The listing builds one solid part. Answer for the finished solid, in the listing's coordinates (mm). A direction names the side the tool comes from. Coordinates: 2 decimals unless noted, no trailing zeros. Order: outer loops, then holes, each group sorted by start corner. A loop starts at its lowest first (then second) coordinate and runs counter-clockwise, first axis right, second up. Notation, with made-up numbers: (63, 61.5) -> (121, 61.5) arc R17 cw to (121, 76.5) -> close; hole circle Ø2 at (-13.5, 76.5). An arc over 180 degrees is marked (long way). Return JSON: item names as keys, results as strings.
from build123d import *

# Parameters (mm, degrees)
SKETCH_1_W          = 73.4
SKETCH_1_H          = 53.4
SKETCH_1_W_2        = 70.4
SKETCH_1_H_2        = 50.4
EXTRUDE_1_DEPTH     = 17
SKETCH_2_W          = 73.4
SKETCH_2_H          = 53.4
EXTRUDE_2_DEPTH     = 1.5
SKETCH_3_W          = 4.5
SKETCH_3_H          = 4.5
EXTRUDE_3_DEPTH     = 10.5
CUT_EXTRUDE_1_REACH = 50.464
SKETCH_4_R          = 2
SKETCH_4_R_2        = 1.7
SKETCH_4_R_3        = 3.75
SKETCH_5_R          = 1
CUT_EXTRUDE_2_DEPTH = 7
SKETCH_6_W          = 71.8
SKETCH_6_H          = 51.8
CUT_EXTRUDE_3_DEPTH = 7
CHAMFER_1_SIZE      = 0.5
CUT_EXTRUDE_4_REACH = 68.988
SKETCH_9_W          = 11
SKETCH_9_H          = 13
CUT_EXTRUDE_5_DEPTH = 0.5


with BuildPart() as part:
    # Эскиз1 → Бобышка-Вытянуть1 (new body)
    with BuildSketch(Plane(origin=(0, 0, 0), x_dir=(1, 0, 0), z_dir=(0, 1, 0))):
        Rectangle(SKETCH_1_W, SKETCH_1_H)
        Rectangle(SKETCH_1_W_2, SKETCH_1_H_2, mode=Mode.SUBTRACT)
    extrude(amount=-EXTRUDE_1_DEPTH)

    # Эскиз2 → Бобышка-Вытянуть2 (add)
    with BuildSketch(Plane(origin=(0, 0, 0), x_dir=(1, 0, 0), z_dir=(0, 1, 0))):
        Rectangle(SKETCH_2_W, SKETCH_2_H)
    extrude(amount=EXTRUDE_2_DEPTH)

    # Эскиз3 → Бобышка-Вытянуть3 (add)
    with BuildSketch(Plane(origin=(0, 0, 0), x_dir=(1, 0, 0), z_dir=(0, 1, 0))):
        with Locations((-32.95, 22.95)):
            Rectangle(SKETCH_3_W, SKETCH_3_H)
        with Locations((32.95, 22.95)):
            Rectangle(SKETCH_3_W, SKETCH_3_H)
        with Locations((-32.95, -22.95)):
            Rectangle(SKETCH_3_W, SKETCH_3_H)
        with Locations((32.95, -22.95)):
            Rectangle(SKETCH_3_W, SKETCH_3_H)
    extrude(amount=-EXTRUDE_3_DEPTH)

    # Эскиз4 → Вырез-Вытянуть1 (cut, up to next)
    with BuildSketch(Plane(origin=(0, 0, 0), x_dir=(1, 0, 0), z_dir=(0, 1, 0)), mode=Mode.PRIVATE) as cut_extrude_1_sk1:
        with Locations(Location((-25.4, -9, 0), (0, 0, 270))):
            Circle(SKETCH_4_R)
    cut_extrude_1_tool1 = extrude(cut_extrude_1_sk1.sketch, amount=CUT_EXTRUDE_1_REACH, mode=Mode.PRIVATE) & part.part
    # Эскиз4 → Вырез-Вытянуть1 (cut, up to next)
    with BuildSketch(Plane(origin=(0, 0, 0), x_dir=(1, 0, 0), z_dir=(0, 1, 0)), mode=Mode.PRIVATE) as cut_extrude_1_sk2:
        with Locations(Location((-12.7, -9, 0), (0, 0, 270))):
            Circle(SKETCH_4_R)
    cut_extrude_1_tool2 = extrude(cut_extrude_1_sk2.sketch, amount=CUT_EXTRUDE_1_REACH, mode=Mode.PRIVATE) & part.part
    # Эскиз4 → Вырез-Вытянуть1 (cut, up to next)
    with BuildSketch(Plane(origin=(0, 0, 0), x_dir=(1, 0, 0), z_dir=(0, 1, 0)), mode=Mode.PRIVATE) as cut_extrude_1_sk3:
        with Locations(Location((0, -9, 0), (0, 0, 270))):
            Circle(SKETCH_4_R)
    cut_extrude_1_tool3 = extrude(cut_extrude_1_sk3.sketch, amount=CUT_EXTRUDE_1_REACH, mode=Mode.PRIVATE) & part.part
    # Эскиз4 → Вырез-Вытянуть1 (cut, up to next)
    with BuildSketch(Plane(origin=(0, 0, 0), x_dir=(1, 0, 0), z_dir=(0, 1, 0)), mode=Mode.PRIVATE) as cut_extrude_1_sk4:
        with Locations(Location((12.7, -9, 0), (0, 0, 270))):
            Circle(SKETCH_4_R)
    cut_extrude_1_tool4 = extrude(cut_extrude_1_sk4.sketch, amount=CUT_EXTRUDE_1_REACH, mode=Mode.PRIVATE) & part.part
    # Эскиз4 → Вырез-Вытянуть1 (cut, up to next)
    with BuildSketch(Plane(origin=(0, 0, 0), x_dir=(1, 0, 0), z_dir=(0, 1, 0)), mode=Mode.PRIVATE) as cut_extrude_1_sk5:
        with Locations(Location((25.4, -9, 0), (0, 0, 270))):
            Circle(SKETCH_4_R)
    cut_extrude_1_tool5 = extrude(cut_extrude_1_sk5.sketch, amount=CUT_EXTRUDE_1_REACH, mode=Mode.PRIVATE) & part.part
    # Эскиз4 → Вырез-Вытянуть1 (cut, up to next)
    with BuildSketch(Plane(origin=(0, 0, 0), x_dir=(1, 0, 0), z_dir=(0, 1, 0)), mode=Mode.PRIVATE) as cut_extrude_1_sk6:
        with Locations(Location((-25.4, 6, 0), (0, 0, 270))):
            Circle(SKETCH_4_R_2)
    cut_extrude_1_tool6 = extrude(cut_extrude_1_sk6.sketch, amount=CUT_EXTRUDE_1_REACH, mode=Mode.PRIVATE) & part.part
    # Эскиз4 → Вырез-Вытянуть1 (cut, up to next)
    with BuildSketch(Plane(origin=(0, 0, 0), x_dir=(1, 0, 0), z_dir=(0, 1, 0)), mode=Mode.PRIVATE) as cut_extrude_1_sk7:
        with Locations(Location((-17.78, 6, 0), (0, 0, 270))):
            Circle(SKETCH_4_R_2)
    cut_extrude_1_tool7 = extrude(cut_extrude_1_sk7.sketch, amount=CUT_EXTRUDE_1_REACH, mode=Mode.PRIVATE) & part.part
    # Эскиз4 → Вырез-Вытянуть1 (cut, up to next)
    with BuildSketch(Plane(origin=(0, 0, 0), x_dir=(1, 0, 0), z_dir=(0, 1, 0)), mode=Mode.PRIVATE) as cut_extrude_1_sk8:
        with Locations(Location((-10.16, 6, 0), (0, 0, 270))):
            Circle(SKETCH_4_R_2)
    cut_extrude_1_tool8 = extrude(cut_extrude_1_sk8.sketch, amount=CUT_EXTRUDE_1_REACH, mode=Mode.PRIVATE) & part.part
    # Эскиз4 → Вырез-Вытянуть1 (cut, up to next)
    with BuildSketch(Plane(origin=(0, 0, 0), x_dir=(1, 0, 0), z_dir=(0, 1, 0)), mode=Mode.PRIVATE) as cut_extrude_1_sk9:
        with Locations(Location((21.5, 8, 0), (0, 0, 270))):
            Circle(SKETCH_4_R_3)
    cut_extrude_1_tool9 = extrude(cut_extrude_1_sk9.sketch, amount=CUT_EXTRUDE_1_REACH, mode=Mode.PRIVATE) & part.part
    add(cut_extrude_1_tool1.solids().sort_by_distance((-25.4, 0, 9))[0], mode=Mode.SUBTRACT)
    add(cut_extrude_1_tool2.solids().sort_by_distance((-12.7, 0, 9))[0], mode=Mode.SUBTRACT)
    add(cut_extrude_1_tool3.solids().sort_by_distance((0, 0, 9))[0], mode=Mode.SUBTRACT)
    add(cut_extrude_1_tool4.solids().sort_by_distance((12.7, 0, 9))[0], mode=Mode.SUBTRACT)
    add(cut_extrude_1_tool5.solids().sort_by_distance((25.4, 0, 9))[0], mode=Mode.SUBTRACT)
    add(cut_extrude_1_tool6.solids().sort_by_distance((-25.4, 0, -6))[0], mode=Mode.SUBTRACT)
    add(cut_extrude_1_tool7.solids().sort_by_distance((-17.78, 0, -6))[0], mode=Mode.SUBTRACT)
    add(cut_extrude_1_tool8.solids().sort_by_distance((-10.16, 0, -6))[0], mode=Mode.SUBTRACT)
    add(cut_extrude_1_tool9.solids().sort_by_distance((21.5, 0, -8))[0], mode=Mode.SUBTRACT)

    # Эскиз5 → Вырез-Вытянуть2 (cut)
    with BuildSketch(Plane.XZ.offset(10.5)):
        with Locations(Location((-33, 23, 0), (0, 0, 270))):
            Circle(SKETCH_5_R)
        with Locations(Location((33, 23, 0), (0, 0, 90))):
            Circle(SKETCH_5_R)
        with Locations(Location((33, -23, 0), (0, 0, 270))):
            Circle(SKETCH_5_R)
        with Locations(Location((-33, -23, 0), (0, 0, 90))):
            Circle(SKETCH_5_R)
    extrude(amount=-CUT_EXTRUDE_2_DEPTH, mode=Mode.SUBTRACT)

    # Эскиз6 → Вырез-Вытянуть3 (cut)
    with BuildSketch(Plane.XZ.offset(17)):
        Rectangle(SKETCH_6_W, SKETCH_6_H)
    extrude(amount=-CUT_EXTRUDE_3_DEPTH, mode=Mode.SUBTRACT)

    # Фаска1
    chamfer_1_edges = [part.edges().sort_by_distance(p)[0] for p in [
        (-36.7, 1.5, 0),
        (0, 1.5, 26.7),
        (36.7, 1.5, 0),
        (0, 1.5, -26.7),
        (-36.7, -7.75, -26.7),
        (36.7, -7.75, -26.7),
        (36.7, -7.75, 26.7),
        (-36.7, -7.75, 26.7),
    ]]
    chamfer(chamfer_1_edges, length=CHAMFER_1_SIZE)

    # Эскиз7 → Вырез-Вытянуть4 (cut, up to next)
    with BuildSketch(Plane(origin=(0, 0, -26.7), x_dir=(-1, 0, 0), z_dir=(0, 0, -1)), mode=Mode.PRIVATE) as cut_extrude_4_sk1:
        with BuildLine():
            Line((-8.3, -13.8), (-8.3, -17))
            Line((-8.3, -17), (-14.7, -17))
            Line((-14.7, -17), (-14.7, -13.8))
            ThreePointArc((-14.7, -13.8), (-11.5, -10.6), (-8.3, -13.8))
        make_face()
    cut_extrude_4_tool1 = extrude(cut_extrude_4_sk1.sketch, amount=-CUT_EXTRUDE_4_REACH, mode=Mode.PRIVATE) & part.part
    # Эскиз7 → Вырез-Вытянуть4 (cut, up to next)
    with BuildSketch(Plane(origin=(0, 0, -26.7), x_dir=(-1, 0, 0), z_dir=(0, 0, -1)), mode=Mode.PRIVATE) as cut_extrude_4_sk2:
        with BuildLine():
            Line((22.2, -13.8), (22.2, -17))
            Line((22.2, -17), (15.8, -17))
            Line((15.8, -17), (15.8, -13.8))
            ThreePointArc((15.8, -13.8), (19, -10.6), (22.2, -13.8))
        make_face()
    cut_extrude_4_tool2 = extrude(cut_extrude_4_sk2.sketch, amount=-CUT_EXTRUDE_4_REACH, mode=Mode.PRIVATE) & part.part
    add(cut_extrude_4_tool1.solids().sort_by_distance((11.5, -14.09872, -26.7))[0], mode=Mode.SUBTRACT)
    add(cut_extrude_4_tool2.solids().sort_by_distance((-19, -14.09872, -26.7))[0], mode=Mode.SUBTRACT)

    # Эскиз9 → Вырез-Вытянуть5 (cut)
    with BuildSketch(Plane(origin=(0, 0, 0), x_dir=(1, 0, 0), z_dir=(0, 1, 0))):
        with Locations((21.5, 8)):
            Rectangle(SKETCH_9_W, SKETCH_9_H)
    extrude(amount=CUT_EXTRUDE_5_DEPTH, mode=Mode.SUBTRACT)


solid = part.part
1. Consider line 1 (X direction, y = -8.25, z = 23); line 2 (Z direction, x = 33, y = -11.75); line 3 (Z direction, x = -10.16, y = 0.4). Determine where each line is inside the solid, lowest interval first. Write a range as from..to.
Answer block:
{"line 1": "x = -36.7..-34, -32..-30.7, 30.7..32, 34..36.7", "line 2": "z = -26.7..-25.9, 25.9..26.7", "line 3": "z = -26.7..-7.7, -4.3..26.7"}
2. Each of these flat-tipped pins is pushed along its axis until it touches: pin 1 Ø3.5 at (x, z) = (22, -6) entering from -Y; pin 2 Ø1.6 at (x, z) = (-33.5, -22.5) entering from -Y; pin 3 Ø8 at (x, z) = (24, 2) entering from -Y; pin 4 Ø2.5 at (x, z) = (-10.16, -6) entering from +Y. Where does it stop, or does it pass through?
Answer block:
{"pin 1": "stops at y = 0.5", "pin 2": "stops at y = -10", "pin 3": "stops at y = 0", "pin 4": "passes through"}
3. The part is cut by section B-B on y = -5.75. Give the vertices of the cut face in (x, z).
Answer block:
{"outline": "(-36.7, -26.2) -> (-36.2, -26.7) -> (36.2, -26.7) -> (36.7, -26.2) -> (36.7, 26.2) -> (36.2, 26.7) -> (-36.2, 26.7) -> (-36.7, 26.2) -> close; hole (-35.2, -20.7) -> (-30.7, -20.7) -> (-30.7, -25.2) -> (30.7, -25.2) -> (30.7, -20.7) -> (35.2, -20.7) -> (35.2, 20.7) -> (30.7, 20.7) -> (30.7, 25.2) -> (-30.7, 25.2) -> (-30.7, 20.7) -> (-35.2, 20.7) -> close; hole circle Ø2 at (-33, -23); hole circle Ø2 at (-33, 23); hole circle Ø2 at (33, -23); hole circle Ø2 at (33, 23)"}
4. The part is cut by section A-A on x = 21.5. Give the vertices of the cut face in (y, z), and give its area (3 significant figures).
Answer block:
{"outline": "(-17, -26.7) -> (1, -26.7) -> (1.5, -26.2) -> (1.5, -11.75) -> (0.5, -11.75) -> (0.5, -14.5) -> (0, -14.5) -> (0, -25.2) -> (-10, -25.2) -> (-10, -25.9) -> (-17, -25.9) -> close; (-17, 25.9) -> (-10, 25.9) -> (-10, 25.2) -> (0, 25.2) -> (0, -1.5) -> (0.5, -1.5) -> (0.5, -4.25) -> (1.5, -4.25) -> (1.5, 26.2) -> (1, 26.7) -> (-17, 26.7) -> close", "area": "107 mm2"}
5. Determine the mould class of faces 1 (the face through (36.7, -8, 0)), 2 (the face through (0, -5, -25.2)), 3 (the face through (-1, -8, -26.7)), 4 (the face through (-26.6, 0.7, 7.4)) for opening direction Z: pulls with the +Z half, pulls with the -Z half, needs draft (parallel to the pull), parting line crosses it, or undercut.
Answer block:
{"face 1": "needs draft", "face 2": "undercut", "face 3": "pulls with the -Z half", "face 4": "undercut"}
6. The part is cut by section C-C on y = -2. Give the vertices of the cut face in (x, z), and give its area (3 significant figures).
Answer block:
{"outline": "(-36.7, -26.2) -> (-36.2, -26.7) -> (36.2, -26.7) -> (36.7, -26.2) -> (36.7, 26.2) -> (36.2, 26.7) -> (-36.2, 26.7) -> (-36.7, 26.2) -> close; hole (-35.2, -20.7) -> (-30.7, -20.7) -> (-30.7, -25.2) -> (30.7, -25.2) -> (30.7, -20.7) -> (35.2, -20.7) -> (35.2, 20.7) -> (30.7, 20.7) -> (30.7, 25.2) -> (-30.7, 25.2) -> (-30.7, 20.7) -> (-35.2, 20.7) -> close", "area": "452 mm2"}
7. The part is cut by section D-D on z = -19. Give the vertices of the cut face in (x, y), and give its area (3 significant figures).
Answer block:
{"outline": "(-36.7, -17) -> (-35.9, -17) -> (-35.9, -10) -> (-35.2, -10) -> (-35.2, 0) -> (35.2, 0) -> (35.2, -10) -> (35.9, -10) -> (35.9, -17) -> (36.7, -17) -> (36.7, 1) -> (36.2, 1.5) -> (-36.2, 1.5) -> (-36.7, 1) -> close", "area": "151 mm2"}
8. For faces 5 (the face through (-1, 1.5, 0)), 6 (the face through (-34, -7, -23)), determine the directions among +Z, -Z, +X, -X, +Y, -Y from which every point of the face is accessible in a straight line to the end or side of a thin tool.
Answer block:
{"face 5": "+Z, -Z, +X, -X, +Y", "face 6": "-Y"}
